For this review, take the finished solid that the model builds, in its own axes (mm). Face numbers are marked on the shaded views. A direction names the side the tool comes from. Coordinates: 2 decimals unless noted, no trailing zeros. Write each loop counter-clockwise with the first axis right and the second up, starting at its lowest first coordinate (ties: lowest second). Pieces come first, ordered by that corner, then holes. Notation, with made-up numbers: M -4,20 L 52,20 A28 ccw 52,43 Z; hole C 56,60.5 d2. An arc over 180 degrees is marked long. Return JSON: item names as keys, results as strings.
```python
from build123d import *

# Parameters (mm, degrees)
PLAT_W                      = 30
PLAT_H                      = 5
EL_MENT_M_CANO_SOUD_1_DEPTH = 70
ENL_V_MAT_EXTRU_1_DEPTH     = 6
CONG_1_R                    = 3


with BuildPart() as part:
    # plat → Elément mécano-soudé1 (new body)
    with BuildSketch(Plane.YZ.offset(-35)):
        Rectangle(PLAT_W, PLAT_H)
    extrude(amount=EL_MENT_M_CANO_SOUD_1_DEPTH)

    # Esquisse2 → Enlèv. mat.-Extru.1 (cut, through all)
    with BuildSketch(Plane(origin=(0, 0, -2.5), x_dir=(-1, 0, 0), z_dir=(0, 0, -1))):
        with BuildLine():
            Line((-14, -15), (-8, -15))
            Line((-8, -15), (-8, 5))
            ThreePointArc((-8, 5), (-11, 8), (-14, 5))
            Line((-14, 5), (-14, -15))
        make_face()
    extrude(amount=-ENL_V_MAT_EXTRU_1_DEPTH, mode=Mode.SUBTRACT)

    # Congé1
    cong_1_edges = [part.edges().sort_by_distance(p)[0] for p in [
        (35, 15, 0),
        (14, -15, 0),
        (8, -15, 0),
        (35, -15, 0),
        (-35, 15, 0),
        (-35, -15, 0),
    ]]
    fillet(cong_1_edges, radius=CONG_1_R)


solid = part.part
```
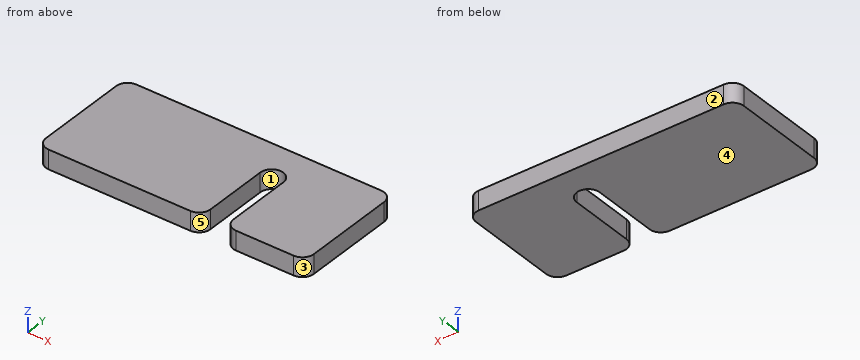
1. For the marked faces 4 and 5, list the 3-axis set-ups (+Z, -Z, +X, -X, +Y, -Y) from which the entire face can be reached by the end or side of a thin tool; tool diameter is ignored.
Checks:
{"face 4": "-Z, +X, -X, +Y, -Y", "face 5": "+Z, -Z, -Y"}
2. Draft analysis for pull direction X (two halves, no side actions). For the marked faces 1, 2 and 3, state which applies: +X half, -X half, draft (parallel to the pull), parting line (faces both ways), or undercut.
Checks:
{"face 1": "undercut", "face 2": "draft", "face 3": "+X half"}
3. We need section C-C (y = -12.75). State the section outline as (x, z) points.
Checks:
{"outline": "M -34.9,-2.5 L 7.9,-2.5 L 7.9,2.5 L -34.9,2.5 Z; M 14.1,-2.5 L 34.9,-2.5 L 34.9,2.5 L 14.1,2.5 Z"}
4. We need section D-D (x = 11). State the section outline as (y, z) points.
Checks:
{"outline": "M 8,-2.5 L 15,-2.5 L 15,2.5 L 8,2.5 Z"}
5. We need section A-A (y = -3.25). State the section outline as (x, z) points.
Checks:
{"outline": "M -35,-2.5 L 8,-2.5 L 8,2.5 L -35,2.5 Z; M 14,-2.5 L 35,-2.5 L 35,2.5 L 14,2.5 Z"}
6. Wall thickness on L1, parallel to X at y = -0.75, z = 1.8; L2, parallel to Y at x = 14.5, z = 1.3; L3, parallel to X at y = 6.25, z = -2.15: over which ranges is each line inside the solid? List them lowest first. Write a range as from..to.
Checks:
{"L1": "-35..8, 14..35", "L2": "-13.66..15", "L3": "-35..8.27, 13.73..35"}
7. We need section B-B (z = 0.9). State the section outline as (x, y) points, plus the area to 3 significant figures.
Checks:
{"outline": "M -35,-12 A3 ccw -32,-15 L 5,-15 A3 ccw 8,-12 L 8,5 A3 cw 14,5 L 14,-12 A3 ccw 17,-15 L 32,-15 A3 ccw 35,-12 L 35,12 A3 ccw 32,15 L -32,15 A3 ccw -35,12 Z", "area": "1,950 mm2"}
